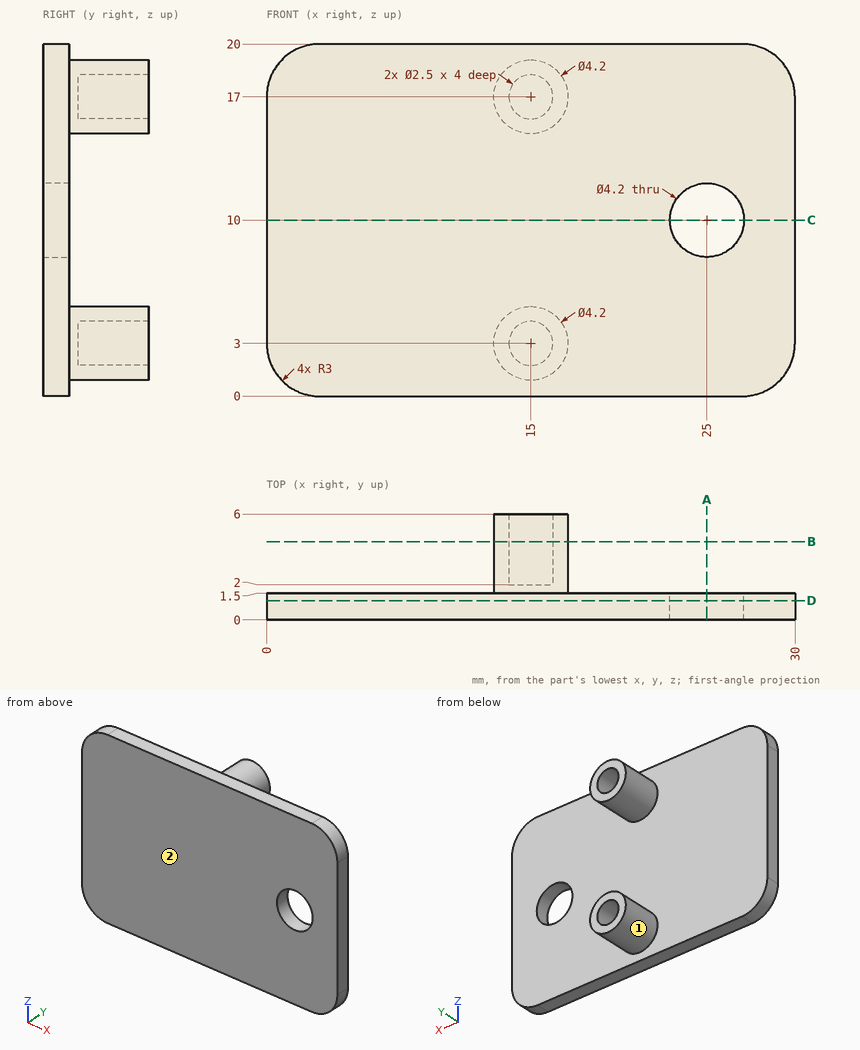
Here's the drawing with two shaded views (mm, measured from the low corner). I have some questions. Coordinates: 2 decimals unless noted, no trailing zeros. Write each loop counter-clockwise with the first axis right and the second up, starting at its lowest first coordinate (ties: lowest second). Pieces come first, ordered by that corner, then holes.
Item 1: If we mould it in two halves opening along Z, with no side actions, what happens to the marked faces 1 and 2? For each: +Z half, -Z half, draft (parallel to the pull), parting line (faces both ways), or undercut.
Item 2: I want a section at A-A on x = 25. Write out the boundary of the cut face in (y, z).
Item 3: Will this pin go through, and if not, where does the flat tip stop? pin 1 (1.5 mm diameter, centred on y = 4, z = 15.5, fed in from +X).
Item 4: I want a section at C-C on z = 10. Write out the boundary of the cut face in (x, y), and give its area (3 significant figures).
Item 5: If I drill on line 1 (X direction, y = 1.25, z = 10); line 2 (Y direction, x = 23.5, z = 19); line 3 (X direction, y = 5.7, z = 17.25), over which ranges is the centre line in solid material (lowest first)?
Item 6: I want a section at D-D on y = 1.1. Write out the boundary of the cut face in (x, z).
Item 7: I want a section at B-B on y = 4.45. Write out the boundary of the cut face in (x, z).
Findings below:
1. face 1: undercut
1. face 2: draft
2. outline: (0, 0) - (1.5, 0) - (1.5, 7.9) - (0, 7.9) - close; (0, 12.1) - (1.5, 12.1) - (1.5, 20) - (0, 20) - close
3. pin 1: stops at x = 16.96
4. outline: (0, 0) - (22.9, 0) - (22.9, 1.5) - (0, 1.5) - close; (27.1, 0) - (30, 0) - (30, 1.5) - (27.1, 1.5) - close
4. area: 38.7 mm2
5. line 1: x = 0 to 22.9, 27.1 to 30
5. line 2: y = 0 to 1.5
5. line 3: x = 12.91 to 13.78, 16.22 to 17.09
6. outline: (0, 3) arc R3 ccw to (3, 0) - (27, 0) arc R3 ccw to (30, 3) - (30, 17) arc R3 ccw to (27, 20) - (3, 20) arc R3 ccw to (0, 17) - close; hole circle Ø4.2 at (25, 10)
7. outline: circle Ø4.2 at (15, 3); circle Ø4.2 at (15, 17); hole circle Ø2.5 at (15, 3); hole circle Ø2.5 at (15, 17)
